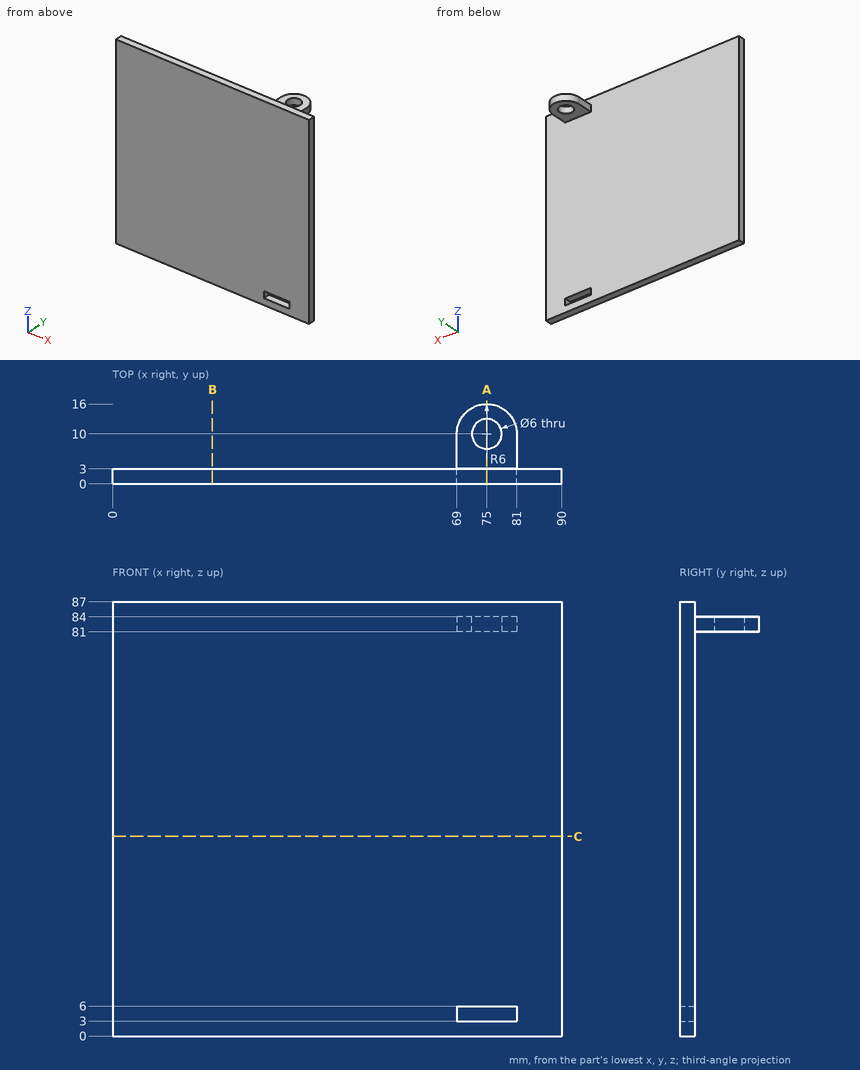
For this review, use the dimensioned drawing (mm, ordinates from the lowest corner) and the shaded views. Give positions to 0.01 mm unless a question says otherwise; leave off trailing zeros. Write each loop counter-clockwise with the first axis right and the second up, starting at its lowest first coordinate (ties: lowest second). Pieces come first, ordered by that corner, then holes. Notation, with made-up numbers: M 6.5,17 L 48.5,17 A21 ccw 48.5,25 Z; hole C 47.5,64.5 d11. An arc over 180 degrees is marked long. Write item = value, one per line. Start each with the question number.
Q1. Clearance check with flat-ended pins moving along their axes: pin 1 (8 mm diameter, centred on x = 75, y = 10, fed in from -Z); pin 2 (9.5 mm diameter, centred on x = 77.5, y = 12.5, fed in from +Z); pin 3 (0.9 mm diameter, centred on y = 7.5, z = 82.5, fed in from +X). State where each tip first meets the part, or that it passes through.
Q2. For line 1 (Y direction, x = 75, z = 83.2); line 2 (Z direction, x = 73.5, y = 1.75); line 3 (Z direction, x = 79.5, y = 8.25), list the stretches that pass through material, from the lowest coordinate up.
Q3. We need section B-B (x = 20). State the section outline as (y, z) points.
Q4. We need section A-A (x = 75). State the section outline as (y, z) points, plus the area to 3 significant figures.
Q5. We need section C-C (z = 40). State the section outline as (x, y) points.
Result set:
q1.pin_1 = 81
q1.pin_2 = 84
q1.pin_3 = 81
q2.line_1 = 0 to 7, 13 to 16
q2.line_2 = 0 to 3, 6 to 87
q2.line_3 = 81 to 84
q3.outline = M 0,0 L 3,0 L 3,87 L 0,87 Z
q4.outline = M 0,0 L 3,0 L 3,3 L 0,3 Z; M 0,6 L 3,6 L 3,81 L 7,81 L 7,84 L 3,84 L 3,87 L 0,87 Z; M 13,81 L 16,81 L 16,84 L 13,84 Z
q4.area = 273 mm2
q5.outline = M 0,0 L 90,0 L 90,3 L 0,3 Z
